Part model, mm, in its own coordinate system. A direction names the side the tool comes from. Round coordinates to 2 decimals unless told otherwise and drop trailing zeros. Order: outer loops, then holes, each group sorted by start corner. A loop starts at its lowest first (then second) coordinate and runs counter-clockwise, first axis right, second up. Notation, with made-up numbers: (-20.75, -4) -> (20.25, -4) arc R32 ccw to (20.25, 35) -> close; hole circle Ø6 at (62, 31.25). An arc over 180 degrees is marked (long way). Use CSV: the item, a comma, the result in double quotes.
```python
from build123d import *

# Parameters (mm, degrees)
BOSS_EXTRUDE1_DEPTH = 5
SKETCH8_W           = 28.13850749
SKETCH8_H           = 12.868219889
CUT_EXTRUDE5_DEPTH  = 10
SKETCH9_R           = 1
CUT_EXTRUDE6_DEPTH  = 1


with BuildPart() as part:
    # Sketch2 → Boss-Extrude1 (new body)
    with BuildSketch(Plane(origin=(0, 0, 0), x_dir=(1, 0, 0), z_dir=(0, 1, 0))):
        Polygon((16.5, 10), (21.5, 6.25), (21.5, 3.75), (16.5, 0), (0, 0), (0, 10), align=None)
    extrude(amount=BOSS_EXTRUDE1_DEPTH)

    # Sketch8 → Cut-Extrude5 (cut)
    with BuildSketch(Plane.XY):
        with Locations((10.578423735, 2.655771349)):
            Rectangle(SKETCH8_W, SKETCH8_H)
        with BuildLine():
            Line((0, 0), (0, 1))
            Line((0, 1), (15.623047352, 1))
            ThreePointArc((15.623047352, 1), (16.450564705, 1.140929202), (17.18478497, 1.547827976))
            Line((17.18478497, 1.547827976), (21.5, 5))
            Line((21.5, 5), (21.5, 4))
            Line((21.5, 4), (17.18478497, 0.547827976))
            ThreePointArc((17.18478497, 0.547827976), (16.450564705, 0.140929202), (15.623047352, 0))
            Line((15.623047352, 0), (0, 0))
        make_face(mode=Mode.SUBTRACT)
    extrude(amount=-CUT_EXTRUDE5_DEPTH, mode=Mode.SUBTRACT)

    # Sketch9 → Cut-Extrude6 (cut)
    with BuildSketch(Plane(origin=(0, 1, 0), x_dir=(1, 0, 0), z_dir=(0, 1, 0))):
        with Locations(Location((7.811523676, 5, 0), (0, 0, 270))):
            Circle(SKETCH9_R)
    extrude(amount=-CUT_EXTRUDE6_DEPTH, mode=Mode.SUBTRACT)


solid = part.part
```
(1) Cut at B-B, the plane x = 7.25. Give the cut face in (y, z), then the cut area to 3 significant figures.
Reply:
outline,"(0, -10) -> (1, -10) -> (1, -5.83) -> (0, -5.83) -> close; (0, -4.17) -> (1, -4.17) -> (1, 0) -> (0, 0) -> close"
area,"8.35 mm2"
(2) Cut at D-D, the plane y = 2.7. Give the cut face in (x, z) (3 decimals), then the cut area to 3 significant figures.
Reply:
outline,"(18.625, -8.406) -> (19.875, -7.469) -> (19.875, -2.531) -> (18.625, -1.594) -> close"
area,"7.34 mm2"
(3) Probe probe 1 along Z at (x, y) = (7.75, 0.85); probe 2 along X at (y, z) = (0.55, -5); probe 3 along Y at (x, z) = (14, -3.25). List the from-to ranges inside material, lowest first. Write a range as [from, to].
Reply:
probe 1,"[-10, -6], [-4, 0]"
probe 2,"[0, 6.81], [8.81, 17.19]"
probe 3,"[0, 1]"
(4) Which spindle directions (+Z, -Z, +X, -X, +Y, -Y) get a long thin tool onto all of the face, cutting with end or side? Do faces 5 (the face through (7.7, 1, -3.8)), 6 (the face through (21.5, 4.5, -5)). Say none if no direction does.
Reply:
face 5,"+Z, -Z, -X, +Y"
face 6,"+Z, -Z, +X, +Y, -Y"
(5) Pull direction X, two halves, no side cores. Call faces 1 (the face through (18.988, 2.389, -8.134)), 2 (the face through (6.835, 0.507, -5.217)), 3 (the face through (8.1, 0.6, -10)), 4 (the face through (0, 0.5, -4.9)): released by +X, released by -X, zero draft, split by the parting line, or undercut.
Reply:
face 1,"released by +X"
face 2,"undercut"
face 3,"zero draft"
face 4,"released by -X"
(6) Cut at C-C, the plane x = 11. Give the cut face in (y, z).
Reply:
outline,"(0, -10) -> (1, -10) -> (1, 0) -> (0, 0) -> close"
(7) Drop flat-ended pins along their axis: P1, Ø4, axis at x = 16.5, z = -5, coming from the -Y side; P2, Ø1, axis at y = 2.5, z = -5, coming from the +X side; P3, Ø2, axis at x = 13.5, y = 2.5, coming from the -Z side; P4, Ø5, axis at x = 7.5, z = -5, coming from the +Y side. Give the stop position or say it passes through.
Reply:
P1,"y = 0"
P2,"x = 20.25"
P3,"through"
P4,"y = 1"
(8) Cut at A-A, the plane z = -5. Give the cut face in (x, y), then the cut area to 3 significant figures.
Reply:
outline,"(0, 0) -> (6.81, 0) -> (6.81, 1) -> (0, 1) -> close; (8.81, 0) -> (15.62, 0) arc R2.5 ccw to (17.18, 0.55) -> (21.5, 4) -> (21.5, 5) -> (17.18, 1.55) arc R2.5 cw to (15.62, 1) -> (8.81, 1) -> close"
area,"19.5 mm2"
